The listing builds one solid part. Answer for the finished solid, in the listing's coordinates (mm). A direction names the side the tool comes from. Give positions to 0.01 mm unless a question says otherwise; leave off trailing zeros. Loops run counter-clockwise (first coordinate to the right, second up) from the corner with the lowest first, then second, coordinate; pieces in that order, holes last. Notation, with made-up numbers: (-13.75, 30) - (6.25, 30) arc R12 ccw to (6.25, 47) - close; hole circle Ø10 at (-19.5, 82.5). An arc over 180 degrees is marked (long way). Write item = value, one per line. Start each with the question number.
1) The part is cut by section A-A on y = 0. Write down the section's boundary in (x, z).
2) The part is cut by section C-C on z = 2.2. Write down the section's boundary in (x, y), plus the area to 3 significant figures.
3) Which of the six approach directions +Z, -Z, +X, -X, +Y, -Y give full straight-line access (tool end or side, diameter ignored) to faces 5 (the flat face through (-21, -2, 6)), 6 (the flat face through (13, -4, 3))?
4) Flat-ended cylindrical pins translate along their axes: P1, Ø2, axis at x = -16.5, y = -19.5, coming from the +Z side; P2, Ø8, axis at x = 0, y = -29, coming from the -Z side. Find the tip coordinate at first contact, or state that the pin passes through.
5) Consider probe 1 along Y at (x, z) = (0, 1.1); probe 2 along Z at (x, y) = (-1, 25); probe 3 along Y at (x, z) = (15, 4.85). Determine where each line is inside the solid, lowest interval first.
6) The mould has two halves that part along X. Classify faces 1 (the cylindrical face through (-10.316, -7.91, 1.521)), 2 (the cylindrical face through (22.4, 7.1, 4.2)), 3 (the cylindrical face through (-4.336, -19.524, 4.232)), 4 (the flat face through (0, -15, 0)): +X half, -X half, draft (parallel to the pull), parting line (faces both ways), or undercut.
7) The part is cut by section D-D on x = -29. Write down the section's boundary in (y, z).
from build123d import *

# Parameters (mm, degrees)
SKETCH1_R           = 35
BOSS_EXTRUDE1_DEPTH = 3
SKETCH2_R           = 13
SKETCH2_R_2         = 3.1
CUT_EXTRUDE1_DEPTH  = 3
SKETCH3_R           = 23.5
SKETCH3_R_2         = 20
BOSS_EXTRUDE2_DEPTH = 3
CHAMFER1_SIZE       = 0.5
CHAMFER2_SIZE       = 0.5


with BuildPart() as part:
    # Sketch1 → Boss-Extrude1 (new body)
    with BuildSketch(Plane.XY):
        Circle(SKETCH1_R)
    extrude(amount=BOSS_EXTRUDE1_DEPTH)

    # Sketch2 → Cut-Extrude1 (cut)
    with BuildSketch(Plane.XY.offset(3)):
        Circle(SKETCH2_R)
        with Locations((0, 29)):
            Circle(SKETCH2_R_2)
        with Locations((29, 0)):
            Circle(SKETCH2_R_2)
        with Locations((0, -29)):
            Circle(SKETCH2_R_2)
        with Locations((-29, 0)):
            Circle(SKETCH2_R_2)
    extrude(amount=-CUT_EXTRUDE1_DEPTH, mode=Mode.SUBTRACT)

    # Sketch3 → Boss-Extrude2 (add)
    with BuildSketch(Plane.XY.offset(3)):
        Circle(SKETCH3_R)
        Circle(SKETCH3_R_2, mode=Mode.SUBTRACT)
    extrude(amount=BOSS_EXTRUDE2_DEPTH)

    # Chamfer1
    chamfer1_edges = [part.edges().sort_by_distance(p)[0] for p in [
        (-23.5, 0, 6),
    ]]
    chamfer(chamfer1_edges, length=CHAMFER1_SIZE)

    # Chamfer2
    chamfer2_edges = [part.edges().sort_by_distance(p)[0] for p in [
        (-20, 0, 6),
    ]]
    chamfer(chamfer2_edges, length=CHAMFER2_SIZE)


solid = part.part
Answer below:
q1.outline = (-35, 0) - (-32.1, 0) - (-32.1, 3) - (-35, 3) - close; (-25.9, 0) - (-13, 0) - (-13, 3) - (-20, 3) - (-20, 5.5) - (-20.5, 6) - (-23, 6) - (-23.5, 5.5) - (-23.5, 3) - (-25.9, 3) - close; (13, 0) - (25.9, 0) - (25.9, 3) - (23.5, 3) - (23.5, 5.5) - (23, 6) - (20.5, 6) - (20, 5.5) - (20, 3) - (13, 3) - close; (32.1, 0) - (35, 0) - (35, 3) - (32.1, 3) - close
q2.outline = circle Ø70 at (0, 0); hole circle Ø6.2 at (-29, 0); hole circle Ø26 at (0, 0); hole circle Ø6.2 at (0, -29); hole circle Ø6.2 at (0, 29); hole circle Ø6.2 at (29, 0)
q2.area = 3,200 mm2
q3.face_5 = +Z, +X, -X, +Y, -Y
q3.face_6 = +Z
q4.P1 = 3
q4.P2 = 0
q5.probe_1 = -35 to -32.1, -25.9 to -13, 13 to 25.9, 32.1 to 35
q5.probe_2 = 0 to 3
q5.probe_3 = -18.09 to -13.23, 13.23 to 18.09
q6.face_1 = undercut
q6.face_2 = parting line
q6.face_3 = undercut
q6.face_4 = draft
q7.outline = (-19.6, 0) - (-3.1, 0) - (-3.1, 3) - (-19.6, 3) - close; (3.1, 0) - (19.6, 0) - (19.6, 3) - (3.1, 3) - close
